Can you work these out from the model? Positions are in its coordinate system, mm. Face numbers are marked on the shaded views. Give positions to 0.01 mm unless a question says otherwise; leave off trailing zeros. Loops run counter-clockwise (first coordinate to the right, second up) from the corner with the lowest first, then second, coordinate; pieces in that order, holes last. Notation, with made-up numbers: (-26.5, 88) - (-21.5, 88) arc R20 cw to (-21.5, 110) - close; hole circle Ø4 at (64.25, 20.25). An arc over 180 degrees is marked (long way). Answer as a JSON object with one key per item and string values.
```python
from build123d import *

# Parameters (mm, degrees)
F0_R     = 6.5
F0_R_2   = 1
F1_DEPTH = 1.5
F2_R     = 2
F2_R_2   = 1
F3_DEPTH = 3.8
F4_R     = 0.6498381819
F5_DEPTH = 1.5


# Not quite as in the source:
# - a feature names something its author has since deleted; it is built from what else it names


with BuildPart() as f1:
    # F0 (on Top) → F1 (new body)
    with BuildSketch(Plane.XY):
        Circle(F0_R)
        Circle(F0_R_2, mode=Mode.SUBTRACT)
    extrude(amount=F1_DEPTH)

    # F2 (on face) → F3 (join)
    with BuildSketch(Plane.XY.offset(1.5)):
        Circle(F2_R)
        Circle(F2_R_2, mode=Mode.SUBTRACT)
    extrude(amount=F3_DEPTH)

    # F4 (on Top) → F5 (cut, through all)
    with BuildSketch(Plane.XY):
        with Locations((0, -3.5616646055)):
            Circle(F4_R)
    extrude(amount=F5_DEPTH, mode=Mode.SUBTRACT)


solid = f1.part
```
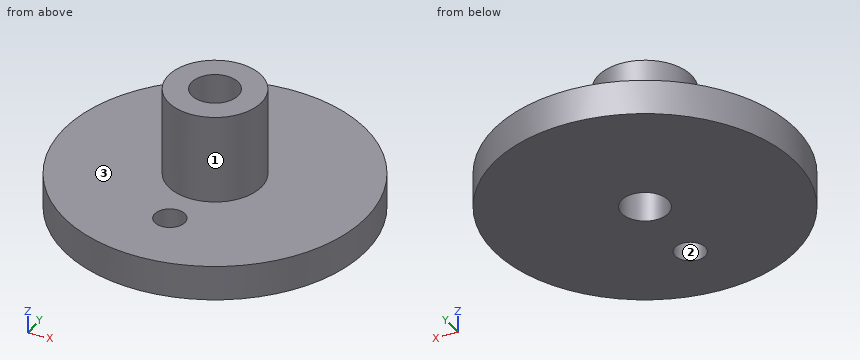
1) Imagine slicing it at A-A on x = 0. Write out the boundary of the cut face in (y, z).
Check sheet entries:
{"outline": "(-6.5, 0) - (-4.21, 0) - (-4.21, 1.5) - (-6.5, 1.5) - close; (-2.91, 0) - (-1, 0) - (-1, 5.3) - (-2, 5.3) - (-2, 1.5) - (-2.91, 1.5) - close; (1, 0) - (6.5, 0) - (6.5, 1.5) - (2, 1.5) - (2, 5.3) - (1, 5.3) - close"}
2) Imagine slicing it at C-C on z = 1.95. Write out the boundary of the cut face in (x, y).
Check sheet entries:
{"outline": "circle Ø4 at (0, 0); hole circle Ø2 at (0, 0)"}
3) I need wall thicknesses on L1, parallel to Y at x = 0, z = 0.3; L2, parallel to Z at x = 5.75, y = 2; L3, parallel to Y at x = -0.5, z = 1.8. Which ranges of each line are inside material? Lowest first, please.
Check sheet entries:
{"L1": "-6.5 to -4.21, -2.91 to -1, 1 to 6.5", "L2": "0 to 1.5", "L3": "-1.94 to -0.87, 0.87 to 1.94"}
4) I'm going to push flat-ended pins straight in: P1, Ø1.5, axis at x = 1.5, z = 4, coming from the -Y side; P2, Ø3, axis at y = -1.5, z = 2.5, coming from the -X side; P3, Ø1.5, axis at x = 3.5, y = -2, coming from the +Z side; P4, Ø1.2, axis at x = 0, y = 0, coming from the -Z side. Where does each tip first touch, or does it pass through?
Check sheet entries:
{"P1": "y = -1.85", "P2": "x = -6.49", "P3": "z = 1.5", "P4": "through"}
5) Imagine slicing it at B-B on y = 0. Write out the boundary of the cut face in (x, z).
Check sheet entries:
{"outline": "(-6.5, 0) - (-1, 0) - (-1, 5.3) - (-2, 5.3) - (-2, 1.5) - (-6.5, 1.5) - close; (1, 0) - (6.5, 0) - (6.5, 1.5) - (2, 1.5) - (2, 5.3) - (1, 5.3) - close"}
6) If we mould it in two halves opening along X, with no side actions, what happens to the marked faces 1, 2 and 3? For each: released by +X, released by -X, zero draft, split by the parting line, or undercut.
Check sheet entries:
{"face 1": "split by the parting line", "face 2": "undercut", "face 3": "zero draft"}
7) Imagine slicing it at D-D on y = 1.75. Write out the boundary of the cut face in (x, z), and give its area (3 significant figures).
Check sheet entries:
{"outline": "(-6.26, 0) - (6.26, 0) - (6.26, 1.5) - (0.97, 1.5) - (0.97, 5.3) - (-0.97, 5.3) - (-0.97, 1.5) - (-6.26, 1.5) - close", "area": "26.1 mm2"}
